```python
from build123d import *

# Parameters (mm, degrees)
SKETCH3_W                = 25.4
SKETCH3_H                = 25.4
SKETCH3_W_2              = 21.336
SKETCH3_H_2              = 21.336
BOSS_EXTRUDE1_DEPTH      = 609.6
BOSS_EXTRUDE1_DEPTH_BACK = 609.6
FILLET1_R                = 3.175
FILLET2_R                = 1.5875
SKETCH4_W                = 25.4
SKETCH4_H                = 50.8
CUT_EXTRUDE1_DEPTH       = 26.4


with BuildPart() as part:
    # Sketch3 → Boss-Extrude1 (new body, two sides)
    with BuildSketch(Plane.XY) as boss_extrude1_sk:
        Rectangle(SKETCH3_W, SKETCH3_H)
        Rectangle(SKETCH3_W_2, SKETCH3_H_2, mode=Mode.SUBTRACT)
    extrude(amount=BOSS_EXTRUDE1_DEPTH)
    extrude(boss_extrude1_sk.sketch, amount=-BOSS_EXTRUDE1_DEPTH_BACK)

    # Fillet1
    fillet1_edges = [part.edges().sort_by_distance(p)[0] for p in [
        (12.7, -12.7, 0),
        (-12.7, -12.7, 0),
        (-12.7, 12.7, 0),
        (12.7, 12.7, 0),
    ]]
    fillet(fillet1_edges, radius=FILLET1_R)

    # Fillet2
    fillet2_edges = [part.edges().sort_by_distance(p)[0] for p in [
        (10.668, -10.668, 0),
        (10.668, 10.668, 0),
        (-10.668, 10.668, 0),
        (-10.668, -10.668, 0),
    ]]
    fillet(fillet2_edges, radius=FILLET2_R)

    # Sketch4 → Cut-Extrude1 (cut, through all)
    with BuildSketch(Plane(origin=(0, 12.7, 0), x_dir=(1, 0, 0), z_dir=(0, 1, 0))):
        with Locations((0, 584.2)):
            Rectangle(SKETCH4_W, SKETCH4_H)
    extrude(amount=-CUT_EXTRUDE1_DEPTH, mode=Mode.SUBTRACT)


solid = part.part
```
For this review, take the finished solid that the model builds, in its own axes (mm). A direction names the side the tool comes from. Round coordinates to 2 decimals unless told otherwise and drop trailing zeros. Write each loop counter-clockwise with the first axis right and the second up, starting at its lowest first coordinate (ties: lowest second). Pieces come first, ordered by that corner, then holes. Notation, with made-up numbers: (78.5, 50.5) - (91.5, 50.5) arc R24 cw to (91.5, 73.5) - close; hole circle Ø5 at (-23, -1.5). An arc over 180 degrees is marked (long way). Answer as a JSON object with one key per item and string values.
1. Tool access review of faces 5 (the face through (11, 0, -558.8)), 6 (the face through (0, 10.668, 34)): name each direction out of +Z, -Z, +X, -X, +Y, -Y from which nothing blocks a thin tool from reaching the whole face with its end or side.
Response values:
{"face 5": "-Z, +X, -X, +Y, -Y", "face 6": "+Z, -Z"}
2. To check wall thickness, follow line 1 along Y through (x, z) = (2.75, -172); line 2 along X through (y, z) = (11.5, 275.5). State the ranges of each line that lie inside material, in increasing order.
Response values:
{"line 1": "y = -12.7 to -10.67, 10.67 to 12.7", "line 2": "x = -12.01 to 12.01"}
3. We need section B-B on x = 3.25. Give the boundary of the cut face in (y, z), then the cut area to 3 significant figures.
Response values:
{"outline": "(-12.7, -558.8) - (-10.67, -558.8) - (-10.67, 609.6) - (-12.7, 609.6) - close; (10.67, -558.8) - (12.7, -558.8) - (12.7, 609.6) - (10.67, 609.6) - close", "area": "4,750 mm2"}
4. Draft analysis for pull direction X (two halves, no side actions). For faces 1 (the face through (0, -10.668, 34)), 2 (the face through (10.668, 0, 34)), 3 (the face through (0, 12.7, 34)), 4 (the face through (-12.7, 0, 34)), state which applies: +X half, -X half, draft (parallel to the pull), parting line (faces both ways), or undercut.
Response values:
{"face 1": "undercut", "face 2": "undercut", "face 3": "draft", "face 4": "-X half"}
